Model file for the job. Use its own axes, mm. Face numbers are marked on the shaded views. Coordinates: 2 decimals unless noted, no trailing zeros. Write each loop counter-clockwise with the first axis right and the second up, starting at its lowest first coordinate (ties: lowest second). Pieces come first, ordered by that corner, then holes. Notation, with made-up numbers: (3, 67.25) - (21, 67.25) arc R16 cw to (21, 74.25) - close; hole circle Ø2 at (82.25, -12). An arc over 180 degrees is marked (long way). Put each result on its own line as item: value. Start each with the question number.
1. Drop a flat-ended pin along its axis: P1, Ø15, axis at x = -13.5, y = -13.5, coming from the +Z side. Give the stop position or say it passes through.
2. Saw through at A-A, the plane x = -33. Write the cut outline in (y, z) (1 decimal), plus the area to 3 significant figures.
3. Drill centre lines: L1, parallel to Y at x = 53.34, z = -1.1 (3 decimals); L2, parallel to Y at x = 6.34, z = -1.95 (3 decimals); L3, parallel to Y at x = 6.34, z = -0.85 (3 decimals). Where is each one in solid material? Low to high. Write a range as from..to.
4. Pull direction X, two halves, no side cores. Call the marked faces 1 and 2: released by +X, released by -X, zero draft, split by the parting line, or undercut.
```python
from build123d import *

# Parameters (mm, degrees)
SKETCH1_W                                     = 139.7
SKETCH1_H                                     = 57.15
BOSS_EXTRUDE1_DEPTH                           = 3.175
SKETCH2_W                                     = 133.35
SKETCH2_H                                     = 50.8
CUT_EXTRUDE1_DEPTH                            = 3.175
FILLET1_R                                     = 12.7
FILLET2_R                                     = 6.35
M2_5X0_45_TAPPED_HOLE1_D                      = 2.05
CSK_FOR_8_FLAT_HEAD_SOCKET_CAP_SCREW1_A_COUNT = 2
CSK_FOR_8_FLAT_HEAD_SOCKET_CAP_SCREW1_A_PITCH = 25.4
CSK_FOR_8_FLAT_HEAD_SOCKET_CAP_SCRE_2_COUNT   = 2
CSK_FOR_8_FLAT_HEAD_SOCKET_CAP_SCRE_2_PITCH   = 31.75
CSK_FOR_8_FLAT_HEAD_SOCKET_CAP_SCRE_3_COUNT   = 2
CSK_FOR_8_FLAT_HEAD_SOCKET_CAP_SCRE_3_PITCH   = 40.659838908
F_4_40_TAPPED_HOLE1_D                         = 2.2606
F_4_40_TAPPED_HOLE1_DEPTH                     = 7.62
F_4_40_TAPPED_HOLE1_TIP                       = 0.679152758
CUT_EXTRUDE2_START                            = -1.5875
CUT_EXTRUDE2_DEPTH                            = 1.5875
MIRROR2_START                                 = -1.5875
MIRROR2_COPY_1_DEPTH                          = 1.5875
FILLET3_R                                     = 6.35
F_8_32_TAPPED_HOLE1_D                         = 3.4544
F_8_32_TAPPED_HOLE1_DEPTH                     = 5.588
F_8_32_TAPPED_HOLE1_TIP                       = 1.037806461


with BuildPart() as part:
    # Sketch1 → Boss-Extrude1 (new, symmetric)
    with BuildSketch(Plane.XY):
        Rectangle(SKETCH1_W, SKETCH1_H)
    extrude(amount=BOSS_EXTRUDE1_DEPTH, both=True)

    # Sketch2 → Cut-Extrude1 (cut)
    with BuildSketch(Plane.XY.offset(3.175)):
        Rectangle(SKETCH2_W, SKETCH2_H)
    extrude(amount=-CUT_EXTRUDE1_DEPTH, mode=Mode.SUBTRACT)

    # Fillet1
    fillet1_edges = [part.edges().sort_by_distance(p)[0] for p in [
        (66.675, -25.4, 1.5875),
        (-66.675, -25.4, 1.5875),
        (-66.675, 25.4, 1.5875),
        (66.675, 25.4, 1.5875),
    ]]
    fillet(fillet1_edges, radius=FILLET1_R)

    # Fillet2
    fillet2_edges = [part.edges().sort_by_distance(p)[0] for p in [
        (69.85, -28.575, 0),
        (-69.85, -28.575, 0),
        (-69.85, 28.575, 0),
        (69.85, 28.575, 0),
    ]]
    fillet(fillet2_edges, radius=FILLET2_R)

    # M2.5x0.45 Tapped Hole1 (through all)
    with Locations(Plane.XY):
        with Locations((-53.34, -16), (-53.34, 16), (-6.34, 16), (-6.34, -16), (6.34, 16), (6.34, -16), (53.34, 16), (53.34, -16)):
            Hole(M2_5X0_45_TAPPED_HOLE1_D / 2)

    # Sketch10 → CSK for #8 Flat Head Socket Cap Screw1 (revolve, cut)
    with BuildSketch(Plane(origin=(-12.7, 15.875, 0), x_dir=(0, -1, 0), z_dir=(1, 0, 0))):
        Polygon((0, 0), (0, 3.175), (2.2479, 3.175), (2.2479, 2.658961536), (4.5593, 0), align=None)
    csk_for_8_flat_head_socket_cap_screw1 = revolve(axis=Axis((-12.7, 15.875, 6.35), (0, 0, -1)), mode=Mode.SUBTRACT)

    # CSK for #8 Flat Head Socket Cap Screw1 a: CSK for #8 Flat Head Socket Cap Screw1 ×2
    with Locations(*[(i * CSK_FOR_8_FLAT_HEAD_SOCKET_CAP_SCREW1_A_PITCH, 0, 0) for i in range(1, CSK_FOR_8_FLAT_HEAD_SOCKET_CAP_SCREW1_A_COUNT)]):
        add(csk_for_8_flat_head_socket_cap_screw1, mode=Mode.SUBTRACT)

    # CSK for _8 Flat Head Socket Cap Scre 2: CSK for #8 Flat Head Socket Cap Screw1 ×2
    with Locations(*[(0, -i * CSK_FOR_8_FLAT_HEAD_SOCKET_CAP_SCRE_2_PITCH, 0) for i in range(1, CSK_FOR_8_FLAT_HEAD_SOCKET_CAP_SCRE_2_COUNT)]):
        add(csk_for_8_flat_head_socket_cap_screw1, mode=Mode.SUBTRACT)

    # CSK for _8 Flat Head Socket Cap Scre 3: CSK for #8 Flat Head Socket Cap Screw1 ×2
    with Locations(*[Vector(0.6246950475544243, -0.7808688094430304, 0) * (i * CSK_FOR_8_FLAT_HEAD_SOCKET_CAP_SCRE_3_PITCH) for i in range(1, CSK_FOR_8_FLAT_HEAD_SOCKET_CAP_SCRE_3_COUNT)]):
        add(csk_for_8_flat_head_socket_cap_screw1, mode=Mode.SUBTRACT)

    # #4-40 Tapped Hole1
    with Locations(Plane.XY.offset(3.175)):
        with Locations((-64.77, 22.86), (-64.77, -22.86), (64.77, 22.86), (64.77, -22.86)):
            Hole(F_4_40_TAPPED_HOLE1_D / 2, depth=F_4_40_TAPPED_HOLE1_DEPTH)
            with Locations((0, 0, -(F_4_40_TAPPED_HOLE1_DEPTH + F_4_40_TAPPED_HOLE1_TIP / 2))):  # 118° drill point
                Cone(0, F_4_40_TAPPED_HOLE1_D / 2, F_4_40_TAPPED_HOLE1_TIP, mode=Mode.SUBTRACT)

    # Sketch14 → Cut-Extrude2 (cut)
    with BuildSketch(Plane.XY.offset(CUT_EXTRUDE2_START)):
        with BuildLine():
            Line((-22.225, 15.875), (-22.225, 25.4))
            Line((-22.225, 25.4), (-50.165, 25.4))
            Line((-50.165, 25.4), (-50.165, 16))
            ThreePointArc((-50.165, 16), (-51.09493597, 13.75493597), (-53.34, 12.825))
            Line((-53.34, 12.825), (-66.674384828, 12.825))
            ThreePointArc((-66.674384828, 12.825), (-66.674846206, 12.762500757), (-66.675, 12.7))
            Line((-66.675, 12.7), (-66.675, 0))
            Line((-66.675, 0), (0, 0))
            Line((0, 0), (0, 6.35))
            Line((0, 6.35), (-12.7, 6.35))
            ThreePointArc((-12.7, 6.35), (-19.435192091, 9.139807909), (-22.225, 15.875))
        make_face()
    cut_extrude2 = extrude(amount=CUT_EXTRUDE2_DEPTH, mode=Mode.SUBTRACT)

    # Mirror1: Cut-Extrude2 across plane
    add(cut_extrude2.mirror(Plane.ZX), mode=Mode.SUBTRACT)

    # Mirror2: Cut-Extrude2 across plane
    add(cut_extrude2.mirror(Plane(origin=(0, 0, 0), x_dir=(0, 0, 1), z_dir=(1, 0, 0))), mode=Mode.SUBTRACT)

    # Mirror2 copy 1 sketch → Mirror2 copy 1 (cut)
    with BuildSketch(Plane(origin=(0, 0, 0), x_dir=(-1, 0, 0), z_dir=(0, 0, 1)).offset(MIRROR2_START)):
        with BuildLine():
            Line((-22.225, 15.875), (-22.225, 25.4))
            Line((-22.225, 25.4), (-50.165, 25.4))
            Line((-50.165, 25.4), (-50.165, 16))
            ThreePointArc((-50.165, 16), (-51.09493597, 13.75493597), (-53.34, 12.825))
            Line((-53.34, 12.825), (-66.674384828, 12.825))
            ThreePointArc((-66.674384828, 12.825), (-66.674846206, 12.762500757), (-66.675, 12.7))
            Line((-66.675, 12.7), (-66.675, 0))
            Line((-66.675, 0), (0, 0))
            Line((0, 0), (0, 6.35))
            Line((0, 6.35), (-12.7, 6.35))
            ThreePointArc((-12.7, 6.35), (-19.435192091, 9.139807909), (-22.225, 15.875))
        make_face()
    extrude(amount=MIRROR2_COPY_1_DEPTH, mode=Mode.SUBTRACT)

    # Fillet3
    # the kernel refuses this fillet: 6.35 mm, written as the material it adds along each edge
    with BuildSketch(Plane(origin=(50.165, -25.4, -1.5875), x_dir=(0, 1, 0), z_dir=(0, 0, 1)), Plane(origin=(22.225, 25.4, -1.5875), x_dir=(0, -1, 0), z_dir=(0, 0, 1)), Plane(origin=(-22.225, -25.4, -1.5875), x_dir=(0, 1, 0), z_dir=(0, 0, 1)), Plane(origin=(-50.165, 25.4, -1.5875), x_dir=(0, -1, 0), z_dir=(0, 0, 1))) as fillet3_piece_1:
        with BuildLine():
            CenterArc((FILLET3_R, FILLET3_R), FILLET3_R, 180, 90)
            Line((0, FILLET3_R), (0, 0))
            Line((0, 0), (FILLET3_R, 0))
        make_face()
    extrude(amount=1.5875)
    with BuildSketch(Plane(origin=(66.674384828, -12.825, -1.5875), x_dir=(-1, 0, 0), z_dir=(0, 0, 1)), Plane(origin=(-66.674384828, 12.825, -1.5875), x_dir=(1, 0, 0), z_dir=(0, 0, 1))) as fillet3_piece_2:
        with BuildLine():
            CenterArc((6.349384828, -6.35), FILLET3_R, 90, 90)
            Line((-0.000615172, -6.35), (-0.635615172, -6.35))
            ThreePointArc((-0.635615172, -6.35), (-0.635615172, -0.125), (-0.634969241, 0.00625))
            Line((-0.634969241, 0.00625), (0, 0.635))
            Line((0, 0.635), (6.349384828, 0.635))
            Line((6.349384828, 0.635), (6.349384828, 0))
        make_face()
    extrude(amount=1.5875)
    with BuildSketch(Plane(origin=(66.674384828, 12.825, -1.5875), x_dir=(-1, 0, 0), z_dir=(0, 0, 1)), Plane(origin=(-66.674384828, -12.825, -1.5875), x_dir=(1, 0, 0), z_dir=(0, 0, 1))) as fillet3_piece_3:
        with BuildLine():
            CenterArc((6.349384828, 6.35), FILLET3_R, 180, 90)
            Line((-0.000615172, 6.35), (-0.635615172, 6.35))
            ThreePointArc((-0.635615172, 6.35), (-0.635615172, 0.125), (-0.634969241, -0.00625))
            Line((-0.634969241, -0.00625), (0, -0.635))
            Line((0, -0.635), (6.349384828, -0.635))
            Line((6.349384828, -0.635), (6.349384828, 0))
        make_face()
    extrude(amount=1.5875)
    with BuildSketch(Plane(origin=(50.165, 25.4, -1.5875), x_dir=(0, -1, 0), z_dir=(0, 0, 1)), Plane(origin=(22.225, -25.4, -1.5875), x_dir=(0, 1, 0), z_dir=(0, 0, 1)), Plane(origin=(-50.165, -25.4, -1.5875), x_dir=(0, 1, 0), z_dir=(0, 0, 1)), Plane(origin=(-22.225, 25.4, -1.5875), x_dir=(0, -1, 0), z_dir=(0, 0, 1))) as fillet3_piece_4:
        with BuildLine():
            CenterArc((FILLET3_R, -FILLET3_R), FILLET3_R, 90, 90)
            Line((0, -FILLET3_R), (0, 0))
            Line((0, 0), (FILLET3_R, 0))
        make_face()
    extrude(amount=1.5875)

    # #8-32 Tapped Hole1
    with Locations(Plane(origin=(0, 28.575, 0), x_dir=(-1, 0, 0), z_dir=(0, 1, 0))):
        with Locations((6.35, 0)):
            Hole(F_8_32_TAPPED_HOLE1_D / 2, depth=F_8_32_TAPPED_HOLE1_DEPTH)
            with Locations((0, 0, -(F_8_32_TAPPED_HOLE1_DEPTH + F_8_32_TAPPED_HOLE1_TIP / 2))):  # 118° drill point
                Cone(0, F_8_32_TAPPED_HOLE1_D / 2, F_8_32_TAPPED_HOLE1_TIP, mode=Mode.SUBTRACT)


solid = part.part
```
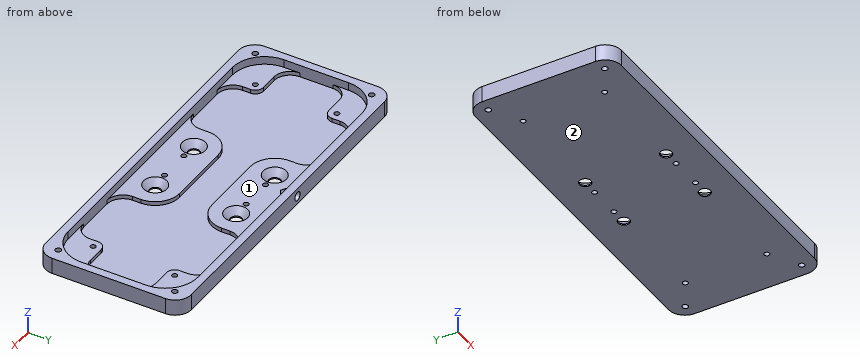
Final values:
1. P1: stops at z = 0
2. outline: (-28.6, -3.2) - (28.6, -3.2) - (28.6, 3.2) - (25.4, 3.2) - (25.4, -1.6) - (-25.4, -1.6) - (-25.4, 3.2) - (-28.6, 3.2) - close
2. area: 121 mm²
3. L1: y = -28.575..-17.025, -14.975..-12.825, 12.825..14.975, 17.025..28.575
3. L2: y = -28.575..-17.025, -14.975..14.975, 17.025..28.575
3. L3: y = -28.575..-17.025, -14.975..-6.35, 6.35..14.975, 17.025..28.575
4. face 1: undercut
4. face 2: zero draft
